```python
from build123d import *

# Parameters (mm, degrees)
BOSS_EXTRUDE1_DEPTH              = 20
SKETCH3_R                        = 26
CUT_EXTRUDE1_DEPTH               = 15
SKETCH4_R                        = 12.5
CUT_EXTRUDE2_DEPTH               = 11.1125
TAP_DRILL_FOR_M6X1_0_TAP2_D      = 5
TAP_DRILL_FOR_M6X1_0_TAP2_DEPTH  = 40
TAP_DRILL_FOR_M6X1_0_TAP2_TIP    = 1.502151548
SKETCH12_W                       = 6
SKETCH12_H                       = 57.3
SKETCH12_W_2                     = 13
CUT_EXTRUDE3_DEPTH               = 20
TAP_DRILL_FOR_M6_HELICOIL1_D     = 6.25
TAP_DRILL_FOR_M6_HELICOIL1_DEPTH = 20
TAP_DRILL_FOR_M6_HELICOIL1_TIP   = 1.877689434
TAP_DRILL_FOR_M6_HELICOIL2_D     = 6.25
TAP_DRILL_FOR_M6_HELICOIL2_DEPTH = 20
TAP_DRILL_FOR_M6_HELICOIL2_TIP   = 1.877689434


with BuildPart() as part:
    # Sketch2 → Boss-Extrude1 (new body)
    with BuildSketch(Plane(origin=(0, 0, 0), x_dir=(0, 0, -1), z_dir=(1, 0, 0))):
        with BuildLine():
            Line((55, -75), (55, 75))
            ThreePointArc((55, 75), (0, 20), (-55, 75))
            Line((-55, 75), (-55, -75))
            Line((-55, -75), (55, -75))
        make_face()
        with BuildLine():
            ThreePointArc((-55, 75), (0, 20), (55, 75))
            Line((55, 75), (-55, 75))
        make_face()
        with BuildLine():
            Line((-55, 75), (55, 75))
            ThreePointArc((55, 75), (0, 130), (-55, 75))
        make_face()
    extrude(amount=BOSS_EXTRUDE1_DEPTH)

    # Sketch3 → Cut-Extrude1 (cut)
    with BuildSketch(Plane(origin=(20, 0, 0), x_dir=(0, 0, -1), z_dir=(1, 0, 0))):
        with Locations((0, 75)):
            Circle(SKETCH3_R)
    extrude(amount=-CUT_EXTRUDE1_DEPTH, mode=Mode.SUBTRACT)

    # Sketch4 → Cut-Extrude2 (cut)
    with BuildSketch(Plane(origin=(5, 0, 0), x_dir=(0, 0, -1), z_dir=(1, 0, 0))):
        with Locations((0, 75)):
            Circle(SKETCH4_R)
    extrude(amount=-CUT_EXTRUDE2_DEPTH, mode=Mode.SUBTRACT)

    # Tap Drill for M6x1.0 Tap2
    with Locations(Plane(origin=(0, -75, 0), x_dir=(-1, 0, 0), z_dir=(0, -1, 0))):
        with Locations((-10, -36.666666667), (-10, -18.333333333), (-10, 0), (-10, 18.333333333), (-10, 36.666666667)):
            Hole(TAP_DRILL_FOR_M6X1_0_TAP2_D / 2, depth=TAP_DRILL_FOR_M6X1_0_TAP2_DEPTH)
            with Locations((0, 0, -(TAP_DRILL_FOR_M6X1_0_TAP2_DEPTH + TAP_DRILL_FOR_M6X1_0_TAP2_TIP / 2))):  # 118° drill point
                Cone(0, TAP_DRILL_FOR_M6X1_0_TAP2_D / 2, TAP_DRILL_FOR_M6X1_0_TAP2_TIP, mode=Mode.SUBTRACT)

    # Sketch12 → Cut-Extrude3 (cut)
    with BuildSketch(Plane(origin=(20, 0, 0), x_dir=(0, 0, -1), z_dir=(1, 0, 0))):
        with Locations((-52, 15)):
            Rectangle(SKETCH12_W, SKETCH12_H)
        with Locations((48.5, 15)):
            Rectangle(SKETCH12_W_2, SKETCH12_H)
    extrude(amount=-CUT_EXTRUDE3_DEPTH, mode=Mode.SUBTRACT)

    # Tap Drill for M6 Helicoil1
    with Locations(Plane(origin=(10, 29.325, 49), x_dir=(1, 0, 0), z_dir=(0, 0, 1))):
        with Locations((0, 0), (0, -28.65)):
            Hole(TAP_DRILL_FOR_M6_HELICOIL1_D / 2, depth=TAP_DRILL_FOR_M6_HELICOIL1_DEPTH)
            with Locations((0, 0, -(TAP_DRILL_FOR_M6_HELICOIL1_DEPTH + TAP_DRILL_FOR_M6_HELICOIL1_TIP / 2))):  # 118° drill point
                Cone(0, TAP_DRILL_FOR_M6_HELICOIL1_D / 2, TAP_DRILL_FOR_M6_HELICOIL1_TIP, mode=Mode.SUBTRACT)

    # Tap Drill for M6 Helicoil2
    with Locations(Plane(origin=(0, 0, -42), x_dir=(-1, 0, 0), z_dir=(0, 0, -1))):
        with Locations((-10, 29.325), (-10, 0.675)):
            Hole(TAP_DRILL_FOR_M6_HELICOIL2_D / 2, depth=TAP_DRILL_FOR_M6_HELICOIL2_DEPTH)
            with Locations((0, 0, -(TAP_DRILL_FOR_M6_HELICOIL2_DEPTH + TAP_DRILL_FOR_M6_HELICOIL2_TIP / 2))):  # 118° drill point
                Cone(0, TAP_DRILL_FOR_M6_HELICOIL2_D / 2, TAP_DRILL_FOR_M6_HELICOIL2_TIP, mode=Mode.SUBTRACT)


solid = part.part
```
Can you work these out from the model? Positions are in its coordinate system, mm. A direction names the side the tool comes from. Give positions to 0.01 mm unless a question says otherwise; leave off trailing zeros. Write each loop counter-clockwise with the first axis right and the second up, starting at its lowest first coordinate (ties: lowest second). Pieces come first, ordered by that corner, then holes. Notation, with made-up numbers: (74.5, 40) - (87.5, 40) arc R17 cw to (87.5, 65) - close; hole circle Ø7 at (27.25, -38.75). An arc over 180 degrees is marked (long way). Write item = value, one per line. Start each with the question number.
1. Thinking about a two-plate mould opening in Z: for faces 1 (the face through (5, 81.1, -11.2)), 2 (the face through (10, 59, -55)), 3 (the face through (10, -13.65, 52)), which applies, released by +Z, released by -Z, zero draft, split by the parting line, or undercut?
2. Please list where these lines run through material, in increasing order: line 1 (Z direction, x = 10, y = -46.5); line 2 (Y direction, x = 3.9, z = 0); line 3 (Y direction, x = 10, z = 41.5).
3. Imagine slicing it at D-D (y = 99). Please give me the cut outline in (x, z).
4. Imagine slicing it at C-C (y = -54.5). Please give me the cut outline in (x, z), and give its area (3 significant figures).
5. For pin 1 (10 mm diameter, centred on x = 13.5, y = 22, fed in from -Z); pin 2 (10 mm diameter, centred on x = 14, z = 22, fed in from +Y); pin 3 (8 mm diameter, centred on x = 10, z = -18.33, fed in from +Y); pin 4 (22.5 mm diameter, centred on y = 75, z = 0, fed in from +X), each with a flat end and sliding along its axis, tell me the tip position at first contact or that it passes through.
6. Imagine slicing it at A-A (x = 18). Please give me the cut outline in (y, z), and give its area (3 significant figures).
7. Imagine slicing it at B-B (z = -45). Please give me the cut outline in (x, y).
8. On a 3-axis mill with a long thin cutter (end or side, diameter ignored), from which of +Z, -Z, +X, -X, +Y, -Y can I reach the whole of each face in a straight line? I mean faces 4 (the face through (9.458, -54.72, -34.226)), 5 (the face through (10, 43.65, -48)), 6 (the face through (10, 60, 55)). Say none if no direction works.
Worked answers:
q1.face_1 = undercut
q1.face_2 = released by -Z
q1.face_3 = zero draft
q2.line_1 = -55 to -39.17, -34.17 to -20.83, -15.83 to -2.5, 2.5 to 15.83, 20.83 to 34.17, 39.17 to 55
q2.line_2 = -75 to 62.5, 87.5 to 130
q2.line_3 = -75 to -2.45, 3.8 to 26.2, 32.45 to 111.09
q3.outline = (0, -49.49) - (20, -49.49) - (20, -10) - (5, -10) - (5, 10) - (20, 10) - (20, 49.49) - (0, 49.49) - close
q4.outline = (0, -55) - (20, -55) - (20, 55) - (0, 55) - close; hole circle Ø5 at (10, -36.67); hole circle Ø5 at (10, -18.33); hole circle Ø5 at (10, 0); hole circle Ø5 at (10, 18.33); hole circle Ø5 at (10, 36.67)
q4.area = 2,100 mm2
q5.pin_1 = -42
q5.pin_2 = 127.31
q5.pin_3 = 128.1
q5.pin_4 = through
q6.outline = (-75, -55) - (-13.65, -55) - (-13.65, -42) - (43.65, -42) - (43.65, -55) - (75, -55) arc R55 ccw to (75, 55) - (43.65, 55) - (43.65, 49) - (-13.65, 49) - (-13.65, 55) - (-75, 55) - close; hole circle Ø52 at (75, 0)
q6.area = 18,000 mm2
q7.outline = (0, -75) - (20, -75) - (20, -13.65) - (0, -13.65) - close; (0, 43.65) - (20, 43.65) - (20, 106.62) - (0, 106.62) - close
q8.face_4 = -Y
q8.face_5 = -Z, +X, -X
q8.face_6 = +Z, +X, -X, +Y, -Y
